Autodesk Inventor part; units mm, degrees
ref_plane "YZ Plane" through (0, 0, 0) normal (1, 0, 0) x (0, 1, 0)
ref_plane "XZ Plane" through (0, 0, 0) normal (0, 1, 0) x (-1, 0, 0)
ref_plane "XY Plane" through (0, 0, 0) normal (0, 0, 1) x (1, 0, 0)
sketch "Boceto1" plane through (0, 0, 0) normal (0, 0, 1) x (1, 0, 0)
  circle A0 centre (0, 0) radius 10.5
  line L0 (8.1551, -6.614) -> (1.0897, -10.4433)
  line L1 (1.0897, -10.4433) -> (-6.614, -8.1551)
  line L2 (-6.614, -8.1551) -> (-10.4433, -1.0897)
  line L3 (-10.4433, -1.0897) -> (-8.1551, 6.614)
  line L4 (-8.1551, 6.614) -> (-1.0897, 10.4433)
  line L5 (-1.0897, 10.4433) -> (6.614, 8.1551)
  line L6 (6.614, 8.1551) -> (10.4433, 1.0897)
  line L7 (10.4433, 1.0897) -> (8.1551, -6.614)
  circle A1 centre (0, 0) radius 5.1
  dimension "d1" = 21
  dimension "d2" = 10.2
extrude "Extrusión1" add sketch "Boceto1" along normal blind 5 contours L7 L0 L1 L2 L3 L4 L5 L6
properties part number "TuercaLlanta"
Work out the finished part from the listing and answer in its coordinate system (mm). Give positions to 0.01 mm unless a question says otherwise; leave off trailing zeros. Loops run counter-clockwise (first coordinate to the right, second up) from the corner with the lowest first, then second, coordinate; pieces in that order, holes last. Notation, with made-up numbers: (89, 30) -> (93, 30) arc R8 ccw to (93, 41) -> close; hole circle Ø11 at (34.25, -14.75). An arc over 180 degrees is marked (long way). Use CSV: the item, a comma, the result in double quotes.
1. The part is cut by section A-A (z = 0.5). Write down the section's boundary in (x, y).
Found:
outline,"(-10.44, -1.09) -> (-6.61, -8.16) -> (1.09, -10.44) -> (8.16, -6.61) -> (10.44, 1.09) -> (6.61, 8.16) -> (-1.09, 10.44) -> (-8.16, 6.61) -> close; hole circle Ø10.2 at (0, 0)"
2. The mould has two halves that part along X. Classify faces 1 (the flat face through (8.502, 4.672, 2.465)), 2 (the flat face through (2, 5, 5)), 3 (the cylindrical face through (2.4, 4.5, 2.5)), 4 (the flat face through (-8.502, -4.672, 2.465)): +X half, -X half, draft (parallel to the pull), parting line (faces both ways), or undercut.
Found:
face 1,"+X half"
face 2,"draft"
face 3,"undercut"
face 4,"-X half"
3. The part is cut by section D-D (y = -6). Write down the section's boundary in (x, z), then the cut area to 3 significant figures.
Found:
outline,"(-7.78, 0) -> (8.34, 0) -> (8.34, 5) -> (-7.78, 5) -> close"
area,"80.6 mm^2"
4. The part is cut by section B-B (x = 0). Write down the section's boundary in (y, z), then the cut area to 3 significant figures.
Found:
outline,"(-10.12, 0) -> (-5.1, 0) -> (-5.1, 5) -> (-10.12, 5) -> close; (5.1, 0) -> (10.12, 0) -> (10.12, 5) -> (5.1, 5) -> close"
area,"50.2 mm^2"
5. Straight lines are drawn through the part: line 1 (Y direction, x = 1, z = 4.5); line 2 (X direction, y = -2, z = 0.85); line 3 (Y direction, x = 0, z = 1.15). For each, find the intervals that lie inside material, in ascending order.
Found:
line 1,"-10.42 to -5, 5 to 9.82"
line 2,"-9.95 to -4.69, 4.69 to 9.53"
line 3,"-10.12 to -5.1, 5.1 to 10.12"
6. The part is cut by section C-C (y = 0.75). Write down the section's boundary in (x, z).
Found:
outline,"(-9.9, 0) -> (-5.04, 0) -> (-5.04, 5) -> (-9.9, 5) -> close; (5.04, 0) -> (10.34, 0) -> (10.34, 5) -> (5.04, 5) -> close"
